Verification items for the finished model (mm, model axes). Face numbers are marked on the shaded views. Round coordinates to 2 decimals unless told otherwise and drop trailing zeros. Write each loop counter-clockwise with the first axis right and the second up, starting at its lowest first coordinate (ties: lowest second). Pieces come first, ordered by that corner, then holes. Notation, with made-up numbers: M -34,62.5 L 10,62.5 A17 ccw 10,72.5 Z; hole C 14,73.5 d9. An arc over 180 degrees is marked long. One line per item, written item: value. Start each with the question number.
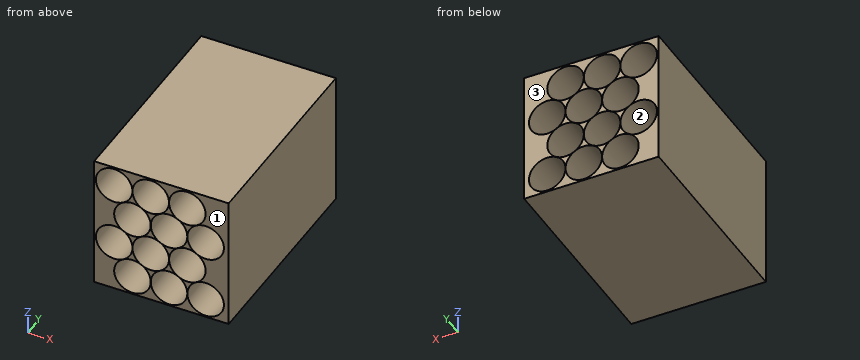
from build123d import *

# Parameters (mm, degrees)
SKETCH1_W               = 97.5
SKETCH1_H               = 97.5
BOSS_EXTRUDE1_DEPTH     = 150
SKETCH5_R               = 13.25
CUT_EXTRUDE5_DEPTH      = 166.085205273
FILL_PATTERN1_OUTLINE_R = 13.25
FILL_PATTERN1_DEPTH     = 150


# Read off the part's stored shape, not the designer's step: Fill Pattern1
with BuildPart() as part:
    # Sketch1 → Boss-Extrude1 (new body)
    with BuildSketch(Plane(origin=(0, 0, 0), x_dir=(1, 0, 0), z_dir=(0, 1, 0))):
        Rectangle(SKETCH1_W, SKETCH1_H)
    extrude(amount=BOSS_EXTRUDE1_DEPTH)

    # Sketch5 → Cut-Extrude5 (cut, through all)
    with BuildSketch(Plane(origin=(0, 150, 0), x_dir=(1, 0, 0), z_dir=(0, 1, 0))):
        with Locations(Location((-34.25, -34.25, 0), (0, 0, 270))):
            Circle(SKETCH5_R)
    extrude(amount=-CUT_EXTRUDE5_DEPTH, mode=Mode.SUBTRACT)

    # Fill Pattern1 outline → Fill Pattern1 (cut)
    with BuildSketch(Plane(origin=(0, 0, 0), x_dir=(1, 0, 0), z_dir=(0, 1, 0))):
        with Locations((32.025, 34.625000363)):
            Circle(FILL_PATTERN1_OUTLINE_R)
        with Locations((32.025, -11.291666546)):
            Circle(FILL_PATTERN1_OUTLINE_R)
        with Locations((18.77, 11.666666909)):
            Circle(FILL_PATTERN1_OUTLINE_R)
        with Locations((5.515, 34.625000363)):
            Circle(FILL_PATTERN1_OUTLINE_R)
        with Locations((18.77, -34.25)):
            Circle(FILL_PATTERN1_OUTLINE_R)
        with Locations((5.515, -11.291666546)):
            Circle(FILL_PATTERN1_OUTLINE_R)
        with Locations((-7.74, 11.666666909)):
            Circle(FILL_PATTERN1_OUTLINE_R)
        with Locations((-20.995, 34.625000363)):
            Circle(FILL_PATTERN1_OUTLINE_R)
        with Locations((-7.74, -34.25)):
            Circle(FILL_PATTERN1_OUTLINE_R)
        with Locations((-20.995, -11.291666546)):
            Circle(FILL_PATTERN1_OUTLINE_R)
        with Locations((-34.25, 11.666666909)):
            Circle(FILL_PATTERN1_OUTLINE_R)
    extrude(amount=FILL_PATTERN1_DEPTH, mode=Mode.SUBTRACT)


solid = part.part
1) Mould release check, pull along Y, two halves, no side actions. Record for the marked faces 1, 2 and 3: pulls with the +Y half, pulls with the -Y half, needs draft (parallel to the pull), parting line crosses it, or undercut.
2) Thickness scan on line 1 (X direction, y = 54, z = -31); line 2 (X direction, y = 105, z = 32.5); line 3 (Z direction, x = -9.5, y = 142.5). Record the ranges inside material, lowest first.
3) Cross-section at B-B (x = -11). Record the boundary of the cut face in (y, z).
4) Cross-section at D-D (z = -32). Record the boundary of the cut face in (x, y).
5) Cross-section at A-A (z = 34.25). State how many separate pieces and enclosed holes the cut face has, then the cut area to 3 significant figures.
Results below:
1. face 1: pulls with the -Y half
1. face 2: needs draft
1. face 3: pulls with the +Y half
2. line 1: x = -48.75 to -33.74, -8.25 to -7.23, 18.26 to 19.28, 44.77 to 48.75
2. line 2: x = -48.75 to -47.38, -21.12 to -20.87, 5.39 to 5.64, 31.9 to 48.75
2. line 3: z = -48.75 to -41.21, -28.04 to -24.8, 1.47 to 4.7, 17.88 to 21.12, 47.38 to 48.75
3. outline: M 0,-48.75 L 150,-48.75 L 150,-43.32 L 0,-43.32 Z; M 0,-25.93 L 150,-25.93 L 150,-24.51 L 0,-24.51 Z; M 0,1.18 L 150,1.18 L 150,2.59 L 0,2.59 Z; M 0,19.99 L 150,19.99 L 150,21.41 L 0,21.41 Z; M 0,47.09 L 150,47.09 L 150,48.75 L 0,48.75 Z
4. outline: M -48.75,0 L -33.98,0 L -33.98,150 L -48.75,150 Z; M -8.01,0 L -7.47,0 L -7.47,150 L -8.01,150 Z; M 18.5,0 L 19.04,0 L 19.04,150 L 18.5,150 Z; M 45.01,0 L 48.75,0 L 48.75,150 L 45.01,150 Z
5. separate pieces: 4
5. enclosed holes: 0
5. area: 2,700 mm²
